```python
from build123d import *

# Parameters (mm, degrees)
REVOLVE_1_ANGLE           = 120.00000000000027
REVOLVE_2_ANGLE           = 30.000000000000068
REVOLVE_2_OTHER_WAY_ANGLE = 30.000000000000068


with BuildPart() as part:
    # Эскиз1 → Повернуть1 (revolve)
    with BuildSketch(Plane(origin=(0, 0, 0), x_dir=(0, 0, -1), z_dir=(1, 0, 0))):
        Polygon((-2e-17, 41.7), (-4.23e-15, 40.5), (95, 40.5), (95, 41.70000000000002), align=None)
    revolve(axis=Axis((0, 0, 0), (0, 0, -1)), revolution_arc=REVOLVE_1_ANGLE)

    # Эскиз3 → Повернуть2 (revolve)
    with BuildSketch(Plane(origin=(0, 0, 0), x_dir=(0, 0, 1), z_dir=(0.499999999999998, -0.8660254037844398, 0))):
        Polygon((-95, -40.500000000000014), (-215, -40.50000000000003), (-215, -41.70000000000003), (-95, -41.700000000000024), align=None)
    revolve(axis=Axis((0, 0, -95), (0, 0, 1)), revolution_arc=REVOLVE_2_ANGLE)

    # Эскиз3 → Повернуть2 other way (revolve)
    with BuildSketch(Plane(origin=(0, 0, 0), x_dir=(0, 0, 1), z_dir=(0.499999999999998, -0.8660254037844398, 0))):
        Polygon((-95, -40.500000000000014), (-215, -40.50000000000003), (-215, -41.70000000000003), (-95, -41.700000000000024), align=None)
    revolve(axis=Axis((0, 0, -95), (0, 0, -1)), revolution_arc=REVOLVE_2_OTHER_WAY_ANGLE)


solid = part.part
```
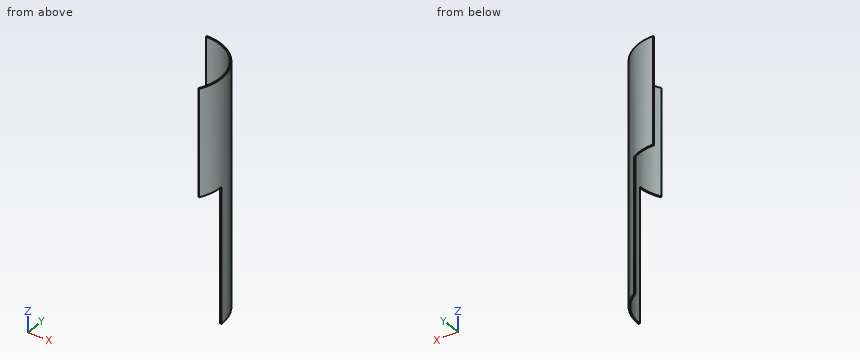
Geometry: final body of the model. Coordinates: model frame, mm. Round coordinates to 2 decimals unless told otherwise and drop trailing zeros. Order: outer loops, then holes, each group sorted by start corner. A loop starts at its lowest first (then second) coordinate and runs counter-clockwise, first axis right, second up. Notation, with made-up numbers: (9, 61) - (48, 61) arc R28 cw to (48, 80) - close; hole circle Ø9 at (77, 51.25). An arc over 180 degrees is marked (long way). Use CSV: the item, a comma, the result in double quotes. Start each with the question number.
Q1. Material intervals for line 1 along Y through (x, z) = (24, -193); line 2 along X through (y, z) = (23.5, -13); line 3 along X through (y, z) = (22, -182), sorted ascending. Write a range as from..to.
Q2. Section query A-A (z = -74). Return loops of the section in (x, y), and give its area (3 significant figures).
Q3. First-contact query: pin 1 (5 mm diameter, centred on x = 35, z = -163.5, fed in from -Y); pin 2 (3 mm diameter, centred on x = 24.5, z = -188, fed in from -Y); pin 3 (1.3 mm diameter, centred on x = 41.5, z = -166, fed in from -Y). Flat tips, straight axial feed; report the tip coordinate or a pass-through.
Q4. Section query B-B (x = 26). Return loops of the section in (y, z).
Result set:
1,line 1,"y = 32.62..34.1"
1,line 2,"x = 32.98..34.45"
1,line 3,"x = 34..35.42"
2,outline,"(0, 40.5) arc R40.5 cw to (35.07, -20.25) - (36.11, -20.85) arc R41.7 ccw to (0, 41.7) - close"
2,area,"103 mm2"
3,pin 1,"stops at y = 15.3"
3,pin 2,"stops at y = 31.05"
3,pin 3,"stops at y = 0"
4,outline,"(31.05, -215) - (32.6, -215) - (32.6, 0) - (31.05, 0) - close"
